from build123d import *

# Parameters (mm, degrees)
SKETCH_1_W      = 120
SKETCH_1_H      = 100
EXTRUDE_1_DEPTH = 10
SKETCH_2_R      = 25
EXTRUDE_2_DEPTH = 100
SKETCH_3_W      = 60
SKETCH_3_H      = 80
EXTRUDE_3_DEPTH = 5
EXTRUDE_4_DEPTH = 80
EXTRUDE_5_DEPTH = 80
FILLET_2_R      = 1
FILLET_3_R      = 1
FILLET_4_R      = 1
FILLET_5_R      = 1
FILLET_6_R      = 2


with BuildPart() as part:
    # 草图1 → 凸台-拉伸1 (new body)
    with BuildSketch(Plane(origin=(0, 0, 0), x_dir=(1, 0, 0), z_dir=(0, 1, 0))):
        Rectangle(SKETCH_1_W, SKETCH_1_H)
    extrude(amount=EXTRUDE_1_DEPTH)

    # 草图2 → 凸台-拉伸2 (add)
    with BuildSketch(Plane(origin=(0, 10, 0), x_dir=(1, 0, 0), z_dir=(0, 1, 0))):
        with Locations(Location((0, 0, 0), (0, 0, 270))):
            Circle(SKETCH_2_R)
    extrude(amount=EXTRUDE_2_DEPTH)

    # 草图3 → 凸台-拉伸3 (add)
    with BuildSketch(Plane(origin=(0, 110, 0), x_dir=(1, 0, 0), z_dir=(0, 1, 0))):
        Rectangle(SKETCH_3_W, SKETCH_3_H)
    extrude(amount=EXTRUDE_3_DEPTH)

    # 草图5 → 凸台-拉伸4 (add)
    with BuildSketch(Plane.XY.offset(40)):
        Polygon((-40, 125), (-30, 115), (-30, 110), (-40, 120), align=None)
    extrude(amount=-EXTRUDE_4_DEPTH)

    # 草图6 → 凸台-拉伸5 (add)
    with BuildSketch(Plane.XY.offset(40)):
        Polygon((30, 115), (34.805168411, 119.110453023), (34.805168411, 115), (30, 110), align=None)
    extrude(amount=-EXTRUDE_5_DEPTH)

    # 圆角2
    fillet_2_edges = [part.edges().sort_by_distance(p)[0] for p in [
        (-40, 125, 0),
    ]]
    fillet(fillet_2_edges, radius=FILLET_2_R)

    # 圆角3
    fillet_3_edges = [part.edges().sort_by_distance(p)[0] for p in [
        (34.805168411, 119.110453023, 0),
    ]]
    fillet(fillet_3_edges, radius=FILLET_3_R)

    # 圆角4
    fillet_4_edges = [part.edges().sort_by_distance(p)[0] for p in [
        (-40, 120, 0),
    ]]
    fillet(fillet_4_edges, radius=FILLET_4_R)

    # 圆角5
    fillet_5_edges = [part.edges().sort_by_distance(p)[0] for p in [
        (34.805168411, 115, 0),
    ]]
    fillet(fillet_5_edges, radius=FILLET_5_R)

    # 圆角6
    fillet_6_edges = [part.edges().sort_by_distance(p)[0] for p in [
        (-60, 10, 0),
        (0, 10, 50),
        (60, 10, 0),
        (0, 10, -50),
    ]]
    fillet(fillet_6_edges, radius=FILLET_6_R)


solid = part.part
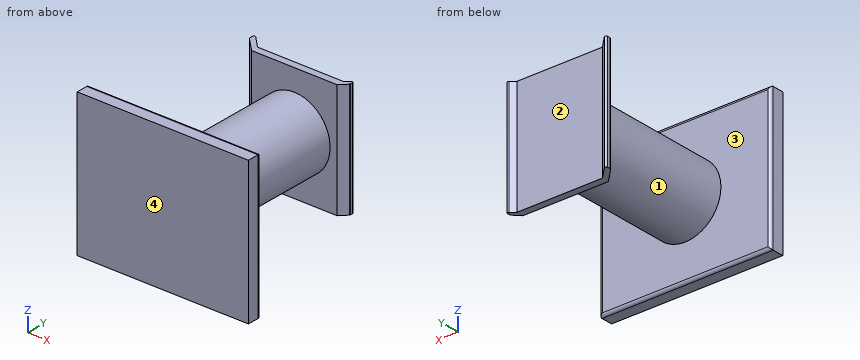
Here's how the part is built. I have some questions about the finished solid (model axes, mm). Face numbers are marked on the shaded views. Coordinates: 2 decimals unless noted, no trailing zeros. Write each loop counter-clockwise with the first axis right and the second up, starting at its lowest first coordinate (ties: lowest second). Pieces come first, ordered by that corner, then holes.
Item 1: I want a section at D-D on x = 0. Write out the boundary of the cut face in (y, z), and give its area (3 significant figures).
Item 2: I want a section at A-A on z = 27. Write out the boundary of the cut face in (x, y), and give its area (3 significant figures).
Item 3: Will these pins go through, and if not, where does the flat tip stop? pin 1 (15 mm diameter, centred on x = 7.5, y = 119, fed in from -Z); pin 2 (12 mm diameter, centred on y = 85, z = -36.5, fed in from +X); pin 3 (1.5 mm diameter, centred on x = -21, z = -1, fed in from +Y); pin 4 (4 mm diameter, centred on x = -2.5, y = 116, fed in from +Z).
Item 4: If I drill on line 1 (Y direction, x = 22, z = 16); line 2 (Y direction, x = -43, z = 42.5); line 3 (Z direction, x = -9, y = 111.5), over which ranges is the centre line in solid material (lowest first)?
Item 5: If we mould it in two halves opening along Y, with no side actions, what happens to the marked faces 1, 2, 3 and 4? For each: +Y half, -Y half, draft (parallel to the pull), parting line (faces both ways), or undercut.
Item 6: I want a section at B-B on x = -35.5. Write out the boundary of the cut face in (y, z).
Item 7: I want a section at C-C on z = 0. Write out the boundary of the cut face in (x, y), and give its area (3 significant figures).
Findings below:
1. outline: (0, -50) - (8, -50) arc R2 ccw to (10, -48) - (10, -25) - (110, -25) - (110, -40) - (115, -40) - (115, 40) - (110, 40) - (110, 25) - (10, 25) - (10, 48) arc R2 ccw to (8, 50) - (0, 50) - close
1. area: 6,400 mm2
2. outline: (-60, 0) - (60, 0) - (60, 8) arc R2 ccw to (58, 10) - (-58, 10) arc R2 ccw to (-60, 8) - close; (-40, 120.41) arc R1 ccw to (-39.71, 119.71) - (-30, 110) - (30, 110) - (34.53, 114.71) arc R1 ccw to (34.81, 115.4) - (34.81, 116.94) arc R1 ccw to (33.16, 117.7) - (30, 115) - (-30, 115) - (-38.29, 123.29) arc R1 ccw to (-40, 122.59) - close
2. area: 1,570 mm2
3. pin 1: stops at z = -40
3. pin 2: passes through
3. pin 3: stops at y = 115
3. pin 4: stops at z = 40
4. line 1: y = 0 to 10, 110 to 115
4. line 2: y = 0 to 10
4. line 3: z = -40 to 40
5. face 1: undercut
5. face 2: +Y half
5. face 3: undercut
5. face 4: -Y half
6. outline: (0, -50) - (8, -50) arc R2 ccw to (10, -48) - (10, 48) arc R2 ccw to (8, 50) - (0, 50) - close; (115.5, -40) - (120.5, -40) - (120.5, 40) - (115.5, 40) - close
7. outline: (-60, 0) - (60, 0) - (60, 8) arc R2 ccw to (58, 10) - (25, 10) - (25, 110) - (30, 110) - (34.53, 114.71) arc R1 ccw to (34.81, 115.4) - (34.81, 116.94) arc R1 ccw to (33.16, 117.7) - (30, 115) - (-30, 115) - (-38.29, 123.29) arc R1 ccw to (-40, 122.59) - (-40, 120.41) arc R1 ccw to (-39.71, 119.71) - (-30, 110) - (-25, 110) - (-25, 10) - (-58, 10) arc R2 ccw to (-60, 8) - close
7. area: 6,570 mm2
